Model file for the job. Use its own axes, mm. Face numbers are marked on the shaded views. A direction names the side the tool comes from. Round coordinates to 2 decimals unless told otherwise and drop trailing zeros. Write each loop counter-clockwise with the first axis right and the second up, starting at its lowest first coordinate (ties: lowest second). Pieces come first, ordered by that corner, then holes.
```python
from build123d import *

# Parameters (mm, degrees)
SKETCH1_W                  = 52
SKETCH1_H                  = 48
BASE_DEPTH                 = 1.04
SKETCH8_W                  = 4.8895
SKETCH8_H                  = 7.6708
DC_POWER_DEPTH             = 3.302
SKETCH9_R                  = 1.25
DC_POWER_HOLE_DEPTH        = 5.842
SKETCH10_R                 = 0.4
DC_POWER_PIN_DEPTH         = 4.1656
SKETCH11_W                 = 2.4638
SKETCH11_H                 = 5.461
PWM_PIN_BASE_DEPTH         = 3.0988
SKETCH12_W                 = 0.635
SKETCH12_H                 = 0.635
PWM_PINS_DEPTH             = 6.0452
SKETCH13_W                 = 6.5278
SKETCH13_H                 = 7.5184
MICRO_HDMI_PORT_DEPTH      = 2.9718
SKETCH14_W                 = 7.5184
SKETCH14_H                 = 5.4102
MICRO_USB_PORT_DEPTH       = 2.54
HEADER_HOLE_REACH          = 74.096
SKETCH15_R                 = 0.8636
SKETCH16_R                 = 1.9939
STANDOFFS_1_DEPTH          = 4.4704
SKETCH17_R                 = 1.9939
SHORT_STANDOFF_DEPTH       = 4.4704
THREADS_IN_STANDOFFS_REACH = 74.096
SKETCH19_R                 = 0.8636
SKETCH20_W                 = 12.1158
SKETCH20_H                 = 12.1158
CPU_DEPTH                  = 1.4732
UART_PLASTIC_DEPTH         = 5.7912
UART_HOLE_DEPTH            = 4.1656
SKETCH23_W                 = 11.5062
SKETCH23_H                 = 5.5372
MICROSD_DEPTH              = 3.302
SKETCH24_W                 = 13.6398
SKETCH24_H                 = 18.2118
EMMC_BOARD_DEPTH           = 1.778
SKETCH25_W                 = 12.319
SKETCH25_H                 = 16.1544
EMMC_CHIP_DEPTH            = 0.7874


with BuildPart() as part:
    # Sketch1 → Base (new body)
    with BuildSketch(Plane(origin=(0, 0, 0), x_dir=(1, 0, 0), z_dir=(0, 1, 0))):
        with Locations((26, 24)):
            Rectangle(SKETCH1_W, SKETCH1_H)
    extrude(amount=BASE_DEPTH)

    # Sketch8 → DC power (add)
    with BuildSketch(Plane(origin=(0, 1.04, 0), x_dir=(1, 0, 0), z_dir=(0, 1, 0))):
        with Locations((16.09725, 44.19)):
            Rectangle(SKETCH8_W, SKETCH8_H)
    extrude(amount=DC_POWER_DEPTH)

    # Sketch9 → DC power hole (cut)
    with BuildSketch(Plane(origin=(0, 0, -48.0254), x_dir=(-1, 0, 0), z_dir=(0, 0, -1))):
        with Locations((-16.09725, 2.3154)):
            Circle(SKETCH9_R)
    extrude(amount=-DC_POWER_HOLE_DEPTH, mode=Mode.SUBTRACT)

    # Sketch10 → DC power pin (add)
    with BuildSketch(Plane(origin=(0, 0, -42.1834), x_dir=(-1, 0, 0), z_dir=(0, 0, -1))):
        with Locations((-16.09725, 2.3154)):
            Circle(SKETCH10_R)
    extrude(amount=DC_POWER_PIN_DEPTH)

    # Sketch11 → PWM pin base (add)
    with BuildSketch(Plane(origin=(0, 1.04, 0), x_dir=(1, 0, 0), z_dir=(0, 1, 0))):
        with Locations((20.9739, 45.2949)):
            Rectangle(SKETCH11_W, SKETCH11_H)
    extrude(amount=PWM_PIN_BASE_DEPTH)

    # Sketch12 → PWM pins (add)
    with BuildSketch(Plane(origin=(0, 4.1388, 0), x_dir=(1, 0, 0), z_dir=(0, 1, 0))):
        with Locations((20.9739, 43.92965)):
            Rectangle(SKETCH12_W, SKETCH12_H)
        with Locations((20.9739, 46.66015)):
            Rectangle(SKETCH12_W, SKETCH12_H)
    extrude(amount=PWM_PINS_DEPTH)

    # Sketch13 → Micro HDMI port (add)
    with BuildSketch(Plane(origin=(0, 1.04, 0), x_dir=(1, 0, 0), z_dir=(0, 1, 0))):
        with Locations((32.8357, 44.6472)):
            Rectangle(SKETCH13_W, SKETCH13_H)
    extrude(amount=MICRO_HDMI_PORT_DEPTH)

    # Sketch14 → Micro USB port (add)
    with BuildSketch(Plane(origin=(0, 1.04, 0), x_dir=(1, 0, 0), z_dir=(0, 1, 0))):
        with Locations((47.5296, 46.1839)):
            Rectangle(SKETCH14_W, SKETCH14_H)
    extrude(amount=MICRO_USB_PORT_DEPTH)

    # Sketch15 → Header hole (cut, up to next)
    with BuildSketch(Plane(origin=(0, 0, 0), x_dir=(-1, 0, 0), z_dir=(0, -1, 0)), mode=Mode.PRIVATE) as header_hole_sk1:
        with Locations(Location((-3, 30.1, 0), (0, 0, 90))):
            Circle(SKETCH15_R)
    header_hole_tool1 = extrude(header_hole_sk1.sketch, amount=-HEADER_HOLE_REACH, mode=Mode.PRIVATE) & part.part
    # Sketch15 → Header hole (cut, up to next)
    with BuildSketch(Plane(origin=(0, 0, 0), x_dir=(-1, 0, 0), z_dir=(0, -1, 0)), mode=Mode.PRIVATE) as header_hole_sk2:
        with Locations(Location((-49, 21.8012, 0), (0, 0, 90))):
            Circle(SKETCH15_R)
    header_hole_tool2 = extrude(header_hole_sk2.sketch, amount=-HEADER_HOLE_REACH, mode=Mode.PRIVATE) & part.part
    # Sketch15 → Header hole (cut, up to next)
    with BuildSketch(Plane(origin=(0, 0, 0), x_dir=(-1, 0, 0), z_dir=(0, -1, 0)), mode=Mode.PRIVATE) as header_hole_sk3:
        with Locations(Location((-40.8, 44.9012, 0), (0, 0, 90))):
            Circle(SKETCH15_R)
    header_hole_tool3 = extrude(header_hole_sk3.sketch, amount=-HEADER_HOLE_REACH, mode=Mode.PRIVATE) & part.part
    add(header_hole_tool1.solids().sort_by_distance((3, 0, -30.1))[0], mode=Mode.SUBTRACT)
    add(header_hole_tool2.solids().sort_by_distance((49, 0, -21.8012))[0], mode=Mode.SUBTRACT)
    add(header_hole_tool3.solids().sort_by_distance((40.8, 0, -44.9012))[0], mode=Mode.SUBTRACT)

    # Sketch16 → Standoffs 1 (add)
    with BuildSketch(Plane.XZ):
        with Locations(Location((49, -21.8012, 0), (0, 0, 270))):
            Circle(SKETCH16_R)
        with Locations(Location((3, -30.1, 0), (0, 0, 270))):
            Circle(SKETCH16_R)
    extrude(amount=STANDOFFS_1_DEPTH)

    # Sketch17 → Short standoff (add)
    with BuildSketch(Plane.XZ):
        with Locations(Location((40.8, -44.9012, 0), (0, 0, 270))):
            Circle(SKETCH17_R)
    extrude(amount=SHORT_STANDOFF_DEPTH)

    # Sketch19 → Threads in standoffs (cut, up to next)
    with BuildSketch(Plane.XZ, mode=Mode.PRIVATE) as threads_in_standoffs_sk1:
        with Locations(Location((40.8, -44.9012, 0), (0, 0, 270))):
            Circle(SKETCH19_R)
    threads_in_standoffs_tool1 = extrude(threads_in_standoffs_sk1.sketch, amount=THREADS_IN_STANDOFFS_REACH, mode=Mode.PRIVATE) & part.part
    # Sketch19 → Threads in standoffs (cut, up to next)
    with BuildSketch(Plane.XZ, mode=Mode.PRIVATE) as threads_in_standoffs_sk2:
        with Locations(Location((49, -21.8012, 0), (0, 0, 270))):
            Circle(SKETCH19_R)
    threads_in_standoffs_tool2 = extrude(threads_in_standoffs_sk2.sketch, amount=THREADS_IN_STANDOFFS_REACH, mode=Mode.PRIVATE) & part.part
    # Sketch19 → Threads in standoffs (cut, up to next)
    with BuildSketch(Plane.XZ, mode=Mode.PRIVATE) as threads_in_standoffs_sk3:
        with Locations(Location((3, -30.1, 0), (0, 0, 270))):
            Circle(SKETCH19_R)
    threads_in_standoffs_tool3 = extrude(threads_in_standoffs_sk3.sketch, amount=THREADS_IN_STANDOFFS_REACH, mode=Mode.PRIVATE) & part.part
    add(threads_in_standoffs_tool1.solids().sort_by_distance((40.8, 0, -44.9012))[0], mode=Mode.SUBTRACT)
    add(threads_in_standoffs_tool2.solids().sort_by_distance((49, 0, -21.8012))[0], mode=Mode.SUBTRACT)
    add(threads_in_standoffs_tool3.solids().sort_by_distance((3, 0, -30.1))[0], mode=Mode.SUBTRACT)

    # Sketch20 → CPU (add)
    with BuildSketch(Plane(origin=(0, 0, 0), x_dir=(-1, 0, 0), z_dir=(0, -1, 0))):
        with Locations((-37.8141, 31.1979)):
            Rectangle(SKETCH20_W, SKETCH20_H)
    extrude(amount=CPU_DEPTH)

    # Sketch21 → UART plastic (add)
    with BuildSketch(Plane(origin=(0, 1.04, 0), x_dir=(1, 0, 0), z_dir=(0, 1, 0))):
        Polygon((52.0254, 38.1254), (47.1994, 38.1254), (47.1994, 27.192440979), (48.636240979, 25.7556), (52.0254, 25.7556), align=None)
    extrude(amount=UART_PLASTIC_DEPTH)

    # Sketch22 → UART hole (cut)
    with BuildSketch(Plane(origin=(0, 6.8312, 0), x_dir=(1, 0, 0), z_dir=(0, 1, 0))):
        Polygon((51.365, 37.465), (49.134996369, 37.465), (47.8598, 36.189803631), (47.8598, 27.465987616), (48.909787616, 26.416), (51.365, 26.416), align=None)
    extrude(amount=-UART_HOLE_DEPTH, mode=Mode.SUBTRACT)

    # Sketch23 → MicroSD (add)
    with BuildSketch(Plane(origin=(0, 1.04, 0), x_dir=(1, 0, 0), z_dir=(0, 1, 0))):
        with Locations((44.8499, 12.6238)):
            Rectangle(SKETCH23_W, SKETCH23_H)
    extrude(amount=MICROSD_DEPTH)

    # Sketch24 → eMMC board (add)
    with BuildSketch(Plane(origin=(0, 1.04, 0), x_dir=(1, 0, 0), z_dir=(0, 1, 0))):
        with Locations((32.1437, 11.1252)):
            Rectangle(SKETCH24_W, SKETCH24_H)
    extrude(amount=EMMC_BOARD_DEPTH)

    # Sketch25 → eMMC chip (add)
    with BuildSketch(Plane(origin=(0, 2.818, 0), x_dir=(1, 0, 0), z_dir=(0, 1, 0))):
        with Locations((32.1437, 10.1219)):
            Rectangle(SKETCH25_W, SKETCH25_H)
    extrude(amount=EMMC_CHIP_DEPTH)


solid = part.part
```
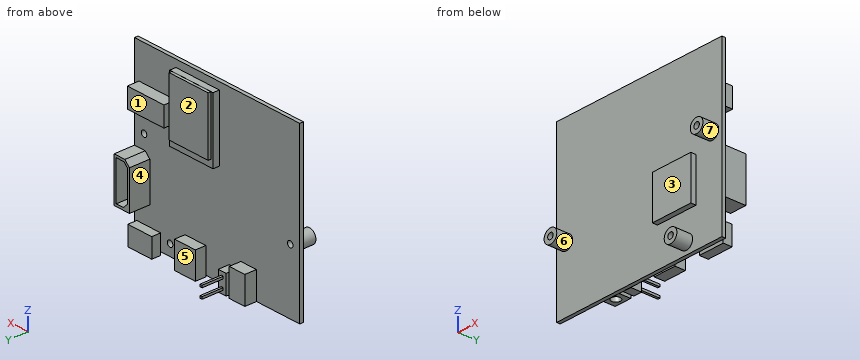
1) Cut at A-A on x = 3. List the corners of the cut face in (y, z).
2) Cut at C-C on x = 40.8. List the corners of the cut face in (y, z), and give its area (3 significant figures).
3) Wall check: probe 1 along Z at (x, y) = (47.5, 1.25); probe 2 along Z at (x, y) = (33.5, 3); probe 3 along X at (y, z) = (1.75, -44). Give the ranges that are in metal, low to high.
4) Flat gauge pins, fed straight in: pin 1 Ø1.5 at (x, y) = (20.5, 6) entering from -Z; pin 2 Ø3 at (x, y) = (39.5, -0.5) entering from -Z; pin 3 Ø1 at (y, z) = (-1.5, -37.5) entering from -X; pin 4 Ø1 at (y, z) = (-2, -41) entering from -X. Where does each tip first touch, or does it go through?
5) Pull direction X, two halves, no side cores. Call the marked faces 5, 6 and 7: released by +X, released by -X, zero draft, split by the parting line, or undercut.
6) Cut at B-B on z = -30.1. List the corners of the cut face in (x, y) (3 decimals).
7) Which spindle directions (+Z, -Z, +X, -X, +Y, -Y) get a long thin tool onto all of the face, cutting with end or side? Do the marked faces 1, 2, 3 and 4. Say none if no direction does.
Result sheet:
1. outline: (-4.47, -32.09) - (0, -32.09) - (0, -48) - (1.04, -48) - (1.04, -30.96) - (-4.47, -30.96) - close; (-4.47, -29.24) - (1.04, -29.24) - (1.04, 0) - (0, 0) - (0, -28.11) - (-4.47, -28.11) - close
2. outline: (-4.47, -46.9) - (0, -46.9) - (0, -48) - (1.04, -48) - (1.04, -45.76) - (-4.47, -45.76) - close; (-4.47, -44.04) - (1.04, -44.04) - (1.04, -15.39) - (4.34, -15.39) - (4.34, -9.86) - (1.04, -9.86) - (1.04, 0) - (0, 0) - (0, -25.14) - (-1.47, -25.14) - (-1.47, -37.26) - (0, -37.26) - (0, -42.91) - (-4.47, -42.91) - close
2. area: 94.4 mm2
3. probe 1: z = -48.89 to -43.48, -38.13 to -26.89, -15.39 to -9.86
3. probe 2: z = -48.41 to -40.89, -18.2 to -2.04
3. probe 3: x = 13.65 to 14.98, 17.21 to 18.54, 19.74 to 22.21, 29.57 to 36.1, 43.77 to 51.29
4. pin 1: stops at z = -46.98
4. pin 2: stops at z = -48
4. pin 3: stops at x = 31.76
4. pin 4: passes through
5. face 5: zero draft
5. face 6: undercut
5. face 7: split by the parting line
6. outline: (0, 0) - (1.006, 0) - (1.006, -4.47) - (2.136, -4.47) - (2.136, 1.04) - (0, 1.04) - close; (3.864, -4.47) - (4.994, -4.47) - (4.994, 0) - (31.756, 0) - (31.756, -1.473) - (43.872, -1.473) - (43.872, 0) - (52, 0) - (52, 1.04) - (52.025, 1.04) - (52.025, 6.831) - (51.365, 6.831) - (51.365, 2.666) - (47.86, 2.666) - (47.86, 6.831) - (47.199, 6.831) - (47.199, 1.04) - (3.864, 1.04) - close
7. face 1: +Z, +X, -X, +Y
7. face 2: +Z, -X, +Y
7. face 3: +Z, +X, -Y
7. face 4: -X, +Y
